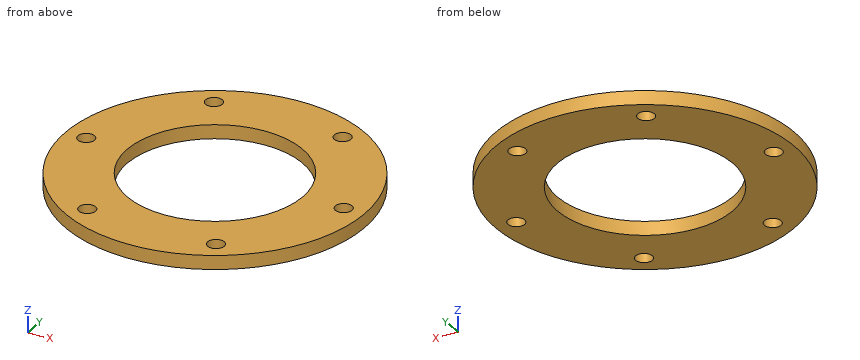
Autodesk Inventor part; units mm, degrees
ref_plane "YZ Plane" through (0, 0, 0) normal (1, 0, 0) x (0, 1, 0)
ref_plane "XZ Plane" through (0, 0, 0) normal (0, 1, 0) x (-1, 0, 0)
ref_plane "XY Plane" through (0, 0, 0) normal (0, 0, 1) x (1, 0, 0)
sketch "Sketch1" plane through (0, 0, 0) normal (0, 0, 1) x (1, 0, 0)
  circle A0 centre (0, 0) radius 63
  circle A1 centre (0, 0) radius 107.5
  dimension "d0" = 126
  dimension "d1" = 215
extrude "Extrusion1" add sketch "Sketch1" against normal blind 10
sketch "Sketch3" plane through (0, 0, 0) normal (0, 0, 1) x (1, 0, 0)
  circle A0 centre (92.5, 0) radius 6
  circle A1 centre (0, 0) radius 92.5 construction
  dimension "d4" = 185
  dimension "d5" = 12
extrude "Cut1" cut sketch "Sketch3" against normal blind 10
pattern_circular "Circular Pattern1" count 6 over 360 about axis through (0, 0, 0) along (0, 0, -1) of "Cut1"
equation "\"d4\" = back_steel_circle_диам_центров"
equation "\"d7\" = Thickness"
equation "\"BendReliefDepth\" = 0.5 * Thickness"
properties part number "NVPH-332 tube flange 1"
Input: part model. Units: mm. Frame: model coordinates. Coordinates: 2 decimals unless noted, no trailing zeros. Loops run counter-clockwise (first coordinate to the right, second up) from the corner with the lowest first, then second, coordinate; pieces in that order, holes last. Notation, with made-up numbers: (9.5, 1.25) -> (66.5, 1.25) arc R21 ccw to (66.5, 31.25) -> close; hole circle Ø8 at (21, 56). An arc over 180 degrees is marked (long way). Use a Markdown table: item, result.
1) Cut plane D-D (z = -1.5). Return the cut outline in (x, y).
Results found:
| item | result |
|---|---|
| outline | circle Ø215 at (0, 0); hole circle Ø12 at (-92.5, 0); hole circle Ø126 at (0, 0); hole circle Ø12 at (-46.25, -80.11); hole circle Ø12 at (-46.25, 80.11); hole circle Ø12 at (46.25, -80.11); hole circle Ø12 at (46.25, 80.11); hole circle Ø12 at (92.5, 0) |
2) Cut plane C-C (y = -56). Return the cut outline in (x, z), then the cut area to 3 significant figures.
Results found:
| item | result |
|---|---|
| outline | (-91.76, -10) -> (-28.86, -10) -> (-28.86, 0) -> (-91.76, 0) -> close; (28.86, -10) -> (91.76, -10) -> (91.76, 0) -> (28.86, 0) -> close |
| area | 1,260 mm2 |
3) Cut plane B-B (y = 0). Return the cut outline in (x, z).
Results found:
| item | result |
|---|---|
| outline | (-107.5, -10) -> (-98.5, -10) -> (-98.5, 0) -> (-107.5, 0) -> close; (-86.5, -10) -> (-63, -10) -> (-63, 0) -> (-86.5, 0) -> close; (63, -10) -> (86.5, -10) -> (86.5, 0) -> (63, 0) -> close; (98.5, -10) -> (107.5, -10) -> (107.5, 0) -> (98.5, 0) -> close |
4) Material intervals for line 1 along X through (y, z) = (85.5, -3.75); line 2 along Y through (x, z) = (51, -5); line 3 along Y through (x, z) = (-49.5, -4), sorted ascending. Write a range as from..to.
Results found:
| item | result |
|---|---|
| line 1 | x = -65.16..-48.88, -43.62..43.62, 48.88..65.16 |
| line 2 | y = -94.63..-83.77, -76.44..-36.99, 36.99..76.44, 83.77..94.63 |
| line 3 | y = -95.43..-85.15, -75.06..-38.97, 38.97..75.06, 85.15..95.43 |
5) Contact query for flat-ended pins moving along their axis: pin 1 (7 mm diameter, centred on x = 92.5, y = 0, fed in from +Z); pin 2 (1.5 mm diameter, centred on y = -84, z = -4.5, fed in from -X); pin 3 (5 mm diameter, centred on x = 44, z = -4, fed in from +Y); pin 4 (3 mm diameter, centred on x = 15, z = -4, fed in from -Y). Output: stop coordinate, or through.
Results found:
| item | result |
|---|---|
| pin 1 | passes through |
| pin 2 | stops at x = -68.01 |
| pin 3 | stops at y = 99.17 |
| pin 4 | stops at y = -106.65 |
6) Cut plane A-A (x = 0). Return the cut outline in (y, z), then the cut area to 3 significant figures.
Results found:
| item | result |
|---|---|
| outline | (-107.5, -10) -> (-63, -10) -> (-63, 0) -> (-107.5, 0) -> close; (63, -10) -> (107.5, -10) -> (107.5, 0) -> (63, 0) -> close |
| area | 890 mm2 |
